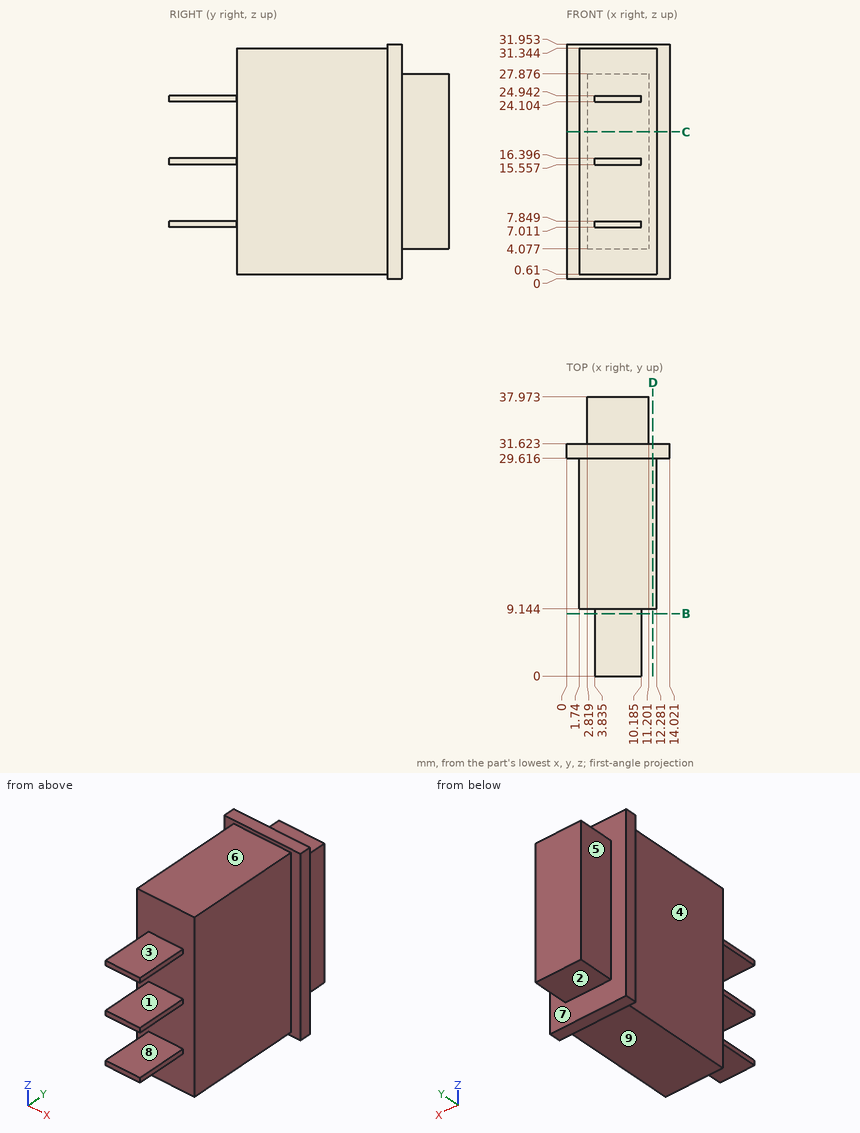
Input: dimensioned drawing with shaded views. Units: mm. Origin: part minimum x, y, z. A direction names the side the tool comes from. Round coordinates to 2 decimals unless told otherwise and drop trailing zeros. Order: outer loops, then holes, each group sorted by start corner. A loop starts at its lowest first (then second) coordinate and runs counter-clockwise, first axis right, second up.
1. Mould query, pull axis Z, two halves, no side actions, for the marked faces 6, 7, 8 and 9. Classes: released by +Z, released by -Z, zero draft, split by the parting line, or undercut.
The answers:
face 6: released by +Z
face 7: zero draft
face 8: undercut
face 9: released by -Z
2. Material intervals for line 1 (Z direction, x = 10.75, y = 29.5); line 2 (X direction, y = 13, z = 19); line 3 (Y direction, x = 7.75, z = 22.5) (1 decimal), sorted ascending.
The answers:
line 1: z = 0.61 to 31.34
line 2: x = 1.74 to 12.28
line 3: y = 9.1 to 38
3. Pin query (flat end, axial travel): P1, Ø3, axis at x = 6, y = 5.5, coming from the +Z side; P2, Ø3, axis at x = 7.5, z = 28.5, coming from the -Y side; P3, Ø2, axis at x = 9.5, y = 20, coming from the +Z side; P4, Ø16.5, axis at y = 22, z = 12.5, coming from the -X side. Return the tip coordinate at first contact, or that it passes through.
The answers:
P1: stops at z = 24.94
P2: stops at y = 9.14
P3: stops at z = 31.34
P4: stops at x = 0
4. Cut plane D-D, the plane x = 11.75. Output: boundary loops of the cut face in (y, z) (1 decimal).
The answers:
outline: (9.1, 0.6) - (29.6, 0.6) - (29.6, 0) - (31.6, 0) - (31.6, 32) - (29.6, 32) - (29.6, 31.3) - (9.1, 31.3) - close
5. Cut plane B-B, the plane y = 8.5. State how many separate pieces and enclosed holes the cut face has.
The answers:
separate pieces: 3
enclosed holes: 0
6. Set-up query: the marked faces 1, 2, 3, 4 and 5. Return all of +Z, -Z, +X, -X, +Y, -Y with unobstructed straight access to the full face (end or side cutting, diameter ignored); none if empty.
The answers:
face 1: +X, -X, -Y
face 2: -Z, +X, -X, +Y
face 3: +Z, +X, -X, -Y
face 4: +Z, -Z, -X, -Y
face 5: +Z, -Z, -X, +Y
7. Cut plane C-C, the plane z = 20. Output: boundary loops of the cut face in (x, y) (1 decimal), then the cut area to 3 significant figures.
The answers:
outline: (0, 29.6) - (1.7, 29.6) - (1.7, 9.1) - (12.3, 9.1) - (12.3, 29.6) - (14, 29.6) - (14, 31.6) - (11.2, 31.6) - (11.2, 38) - (2.8, 38) - (2.8, 31.6) - (0, 31.6) - close
area: 297 mm2
